Autodesk Inventor part; units mm, degrees
ref_plane "YZ Plane" through (0, 0, 0) normal (1, 0, 0) x (0, 1, 0)
ref_plane "XZ Plane" through (0, 0, 0) normal (0, 1, 0) x (-1, 0, 0)
ref_plane "XY Plane" through (0, 0, 0) normal (0, 0, 1) x (1, 0, 0)
sketch "Skizze1" plane through (0, 0, 0) normal (0, 1, 0) x (-1, 0, 0)
  line L0 (-20, 20) -> (20, 20)
  line L1 (20, 20) -> (20, -20)
  line L2 (20, -20) -> (-20, -20)
  line L3 (-20, -20) -> (-20, 20)
  line L4 (-20, 20) -> (20, -20) construction
  line L5 (20, 20) -> (-20, -20) construction
  point P0 (0, 0)
  dimension "d2" = 40
  dimension "d3" = 40
extrude "Extrusion1" add sketch "Skizze1" along normal blind 300
sketch "Skizze2" plane through (20, 0, 20) normal (1, 0, 0) x (0, 0, -1)
  line L0 (0, 0) -> (40, 0)
  point P0 (20, 0)
  point P1 (20, 20)
  point P2 (20, 0)
  dimension "d4" = 20
hole "Bohrung1" at (20, 20, 0) direction (-1, 0, 0) diameter 8 end through all counterbore diameter 18 counterbore depth 10
equation "\"d3\" = d2"
properties part number "Adrian_Cameraarmseiten"
Model file for the job. Use its own axes, mm. A direction names the side the tool comes from. Give positions to 0.01 mm unless a question says otherwise; leave off trailing zeros. Write each loop counter-clockwise with the first axis right and the second up, starting at its lowest first coordinate (ties: lowest second). Pieces come first, ordered by that corner, then holes. Notation, with made-up numbers: (87, 87) -> (133, 87) arc R22 ccw to (133, 114) -> close; hole circle Ø4 at (77.5, -11.75). An arc over 180 degrees is marked (long way). Use CSV: the item, a comma, the result in double quotes. Start each with the question number.
1) Two-plate mould, pull along Y, no slides. Class faces 1 (the flat face through (0, 0, 0)), 2 (the flat face through (20, 148, 0)), 3 (the flat face through (10, 24, -2)): released by +Y, released by -Y, zero draft, split by the parting line, or undercut.
2) Pin check, flat tips, straight feed: P1, Ø14.5, axis at y = 16, z = 4, coming from the +X side; P2, Ø7, axis at y = 20, z = 0, coming from the +X side. Stop position of each tip, or through.
3) Drill centre lines: L1, parallel to Z at x = 14.5, y = 20; L2, parallel to Y at x = 17, z = 0; L3, parallel to Y at x = -5.75, z = 0. Where is each one in solid material? Low to high.
4) Cut at B-B on z = 0. List the corners of the cut face in (x, y), plus the area to 3 significant figures.
5) Cut at A-A on y = 20. List the corners of the cut face in (x, z).
6) Tool access for faces 4 (the cylindrical face through (-5.21, 16.034, 0.521)), 5 (the cylindrical face through (14.93, 28.786, 1.951)): list every direction of +Z, -Z, +X, -X, +Y, -Y with a clear straight run to the whole face (end or side of a thin tool).
Final values:
1,face 1,"released by -Y"
1,face 2,"zero draft"
1,face 3,"undercut"
2,P1,"stops at x = 20"
2,P2,"passes through"
3,L1,"z = -20 to -9, 9 to 20"
3,L2,"y = 0 to 11, 29 to 300"
3,L3,"y = 0 to 16, 24 to 300"
4,outline,"(-20, 0) -> (20, 0) -> (20, 11) -> (10, 11) -> (10, 16) -> (-20, 16) -> close; (-20, 24) -> (10, 24) -> (10, 29) -> (20, 29) -> (20, 300) -> (-20, 300) -> close"
4,area,"11,600 mm2"
5,outline,"(-20, -20) -> (20, -20) -> (20, -9) -> (10, -9) -> (10, -4) -> (-20, -4) -> close; (-20, 4) -> (10, 4) -> (10, 9) -> (20, 9) -> (20, 20) -> (-20, 20) -> close"
6,face 4,"+X, -X"
6,face 5,"+X"
